For this review, take the finished solid that the model builds, in its own axes (mm). A direction names the side the tool comes from. Give positions to 0.01 mm unless a question says otherwise; leave off trailing zeros. Loops run counter-clockwise (first coordinate to the right, second up) from the corner with the lowest first, then second, coordinate; pieces in that order, holes last. Notation, with made-up numbers: (-5.5, 87.5) - (49.5, 87.5) arc R6 ccw to (49.5, 92.5) - close; hole circle Ø7 at (51, 0). An arc over 180 degrees is marked (long way). Use CSV: the item, a comma, the result in double quotes. Start each with the question number.
1. For faces 1 (the flat face through (-4, -2.704, -9)), 2 (the flat face through (-1, -26.204, -15)), 3 (the cylindrical face through (-25.64, -28.65, -14.79)), list the 3-axis set-ups (+Z, -Z, +X, -X, +Y, -Y) from which the entire face can be reached by the end or side of a thin tool; tool diameter is ignored.
2. Mouldability with a two-part tool opening along Y and no side actions: class faces 4 (the flat face through (-1.8, 3.5, 25)), 5 (the flat face through (-14, 37.796, -2)), 6 (the flat face through (-9, 8.296, 1)) as pulls with the +Y half, pulls with the -Y half, needs draft (parallel to the pull), parting line crosses it, or undercut.
3. Take a section at A-A on z = -5.5. Give the boundary of the cut face in (x, y), plus the area to 3 significant figures.
4. Take a section at D-D on x = -6.5. Give the boundary of the cut face in (y, z), plus the area to 3 significant figures.
5. Wall thickness on line 1 (Y direction, x = -15.5, z = 14.5); line 2 (Y direction, x = -5.5, z = -20.5); line 3 (Z direction, x = -25, y = -14): over which ranges is each line inside the solid? List them lowest first.
6. Take a section at C-C on z = -21.5. Give the boundary of the cut face in (x, y).
7. For pin 1 (3 mm diameter, centred on y = 7.5, z = -11.5, fed in from -X); pin 2 (18.5 mm diameter, centred on y = -7.5, z = 17, fed in from -X); pin 3 (4 mm diameter, centred on x = -23, y = 1, fed in from -Z), all flat-tipped, find the tip position at first contact; note any pin that passes through.
8. Take a section at B-B on y = 4.5. Give the boundary of the cut face in (x, z), plus the area to 3 significant figures.
```python
from build123d import *

# Parameters (mm, degrees)
F0_W      = 28
F0_H      = 69
F1_DEPTH  = 25
F2_T      = -2
F3_R      = 5
F4_R      = 10
F5_W      = 6.9
F5_H      = 11
F6_DEPTH  = 25
F7_W      = 2
F7_H      = 45
F8_DEPTH  = 25
F10_W     = 2
F10_H     = 11
F11_DEPTH = 18
F12_DEPTH = 30


with BuildPart() as f1:
    # F0 (on Top) → F1 (new body)
    with BuildSketch(Plane.XY):
        with Locations((-14.1341709197, 3.2960948795)):
            Rectangle(F0_W, F0_H)
    extrude(amount=F1_DEPTH)

    # F2
    f2_openings = [f1.faces().sort_by_distance(p)[0] for p in [
        (-14.134171, 3.296095, 25),
    ]]
    offset(amount=F2_T, openings=f2_openings)

    # F3
    f3_edges = [f1.edges().sort_by_distance(p)[0] for p in [
        (-0.134171, -31.203905, 12.5),
        (-28.134171, -31.203905, 12.5),
        (-0.134171, 37.796095, 12.5),
        (-28.134171, 37.796095, 12.5),
    ]]
    fillet(f3_edges, radius=F3_R)

    # F4
    f4_edges = [f1.edges().sort_by_distance(p)[0] for p in [
        (-26.134171, 35.796095, 13.5),
        (-26.134171, -29.203905, 13.5),
        (-2.134171, -29.203905, 13.5),
        (-2.134171, 35.796095, 13.5),
    ]]
    fillet(f4_edges, radius=F4_R)

    # F5 (on face) → F6 (cut)
    with BuildSketch(Plane.XY.offset(2)):
        with Locations((-8.5841709197, 2.7960948795)):
            Rectangle(F5_W, F5_H)
    extrude(amount=-F6_DEPTH, mode=Mode.SUBTRACT)

    # F7 (on face) → F8 (cut)
    with BuildSketch(Plane.XY.offset(25)):
        with Locations((-27.1341709197, 3.2960948795)):
            Rectangle(F7_W, F7_H)
    extrude(amount=-F8_DEPTH, mode=Mode.SUBTRACT)

    # F10 (on face) → F11 (join)
    with BuildSketch(Plane(origin=(0, 0, 0), x_dir=(1, 0, 0), z_dir=(0, 0, -1))):
        with Locations((-4.1341709197, -2.7960948795)):
            Rectangle(F10_W, F10_H)
    extrude(amount=F11_DEPTH)

    # F10 (on face) → F12 (join)
    with BuildSketch(Plane(origin=(0, 0, 0), x_dir=(1, 0, 0), z_dir=(0, 0, -1))):
        with BuildLine():
            ThreePointArc((-1.6341702342, -32.7960948795), (-2.6592967008, -35.2709690983), (-5.1341709197, -36.296095565))
            Line((-5.1341709197, -36.296095565), (-23.1341709197, -36.296095565))
            ThreePointArc((-23.1341709197, -36.296095565), (-25.6090451385, -35.2709690983), (-26.6341716051, -32.7960948795))
            Line((-26.6341716051, -32.7960948795), (-26.6341716051, -25.7960948795))
            Line((-26.6341716051, -25.7960948795), (-28.1341709197, -25.7960948795))
            Line((-28.1341709197, -25.7960948795), (-28.1341709197, -32.7960948795))
            ThreePointArc((-28.1341709197, -32.7960948795), (-26.6697048256, -36.3316287854), (-23.1341709197, -37.7960948795))
            Line((-23.1341709197, -37.7960948795), (-5.1341709197, -37.7960948795))
            ThreePointArc((-5.1341709197, -37.7960948795), (-1.5986370137, -36.3316287854), (-0.1341709197, -32.7960948795))
            Line((-0.1341709197, -32.7960948795), (-1.6341702342, -32.7960948795))
        make_face()
        with BuildLine():
            Line((-1.6341709197, 26.2039051205), (-0.1341709197, 26.2039051205))
            ThreePointArc((-0.1341709197, 26.2039051205), (-1.5986370137, 29.7394390264), (-5.1341709197, 31.2039051205))
            Line((-5.1341709197, 31.2039051205), (-23.1341709197, 31.2039051205))
            ThreePointArc((-23.1341709197, 31.2039051205), (-26.6697048256, 29.7394390264), (-28.1341709197, 26.2039051205))
            Line((-28.1341709197, 26.2039051205), (-28.1341709197, 19.2039051205))
            Line((-28.1341709197, 19.2039051205), (-26.6341709197, 19.2039051205))
            Line((-26.6341709197, 19.2039051205), (-26.6341709197, 26.2039051205))
            ThreePointArc((-26.6341709197, 26.2039051205), (-25.6090446538, 28.6787788546), (-23.1341709197, 29.7039051205))
            Line((-23.1341709197, 29.7039051205), (-5.1341709197, 29.7039051205))
            ThreePointArc((-5.1341709197, 29.7039051205), (-2.6592971855, 28.6787788546), (-1.6341709197, 26.2039051205))
        make_face()
    extrude(amount=F12_DEPTH)


solid = f1.part
```
Check result:
1,face 1,"-Z, +X, -X"
1,face 2,"-Z, +X"
1,face 3,"-Z"
2,face 4,"needs draft"
2,face 5,"pulls with the +Y half"
2,face 6,"undercut"
3,outline,"(-28.13, -26.2) arc R5 ccw to (-23.13, -31.2) - (-5.13, -31.2) arc R5 ccw to (-0.13, -26.2) - (-1.63, -26.2) arc R3.5 cw to (-5.13, -29.7) - (-23.13, -29.7) arc R3.5 cw to (-26.63, -26.2) - (-26.63, -19.2) - (-28.13, -19.2) - close; (-28.13, 25.8) - (-26.63, 25.8) - (-26.63, 32.8) arc R3.5 cw to (-23.13, 36.3) - (-5.13, 36.3) arc R3.5 cw to (-1.63, 32.8) - (-0.13, 32.8) arc R5 ccw to (-5.13, 37.8) - (-23.13, 37.8) arc R5 ccw to (-28.13, 32.8) - close; (-5.13, -2.7) - (-3.13, -2.7) - (-3.13, 8.3) - (-5.13, 8.3) - close"
3,area,"137 mm²"
4,outline,"(-31.2, -30) - (-29.7, -30) - (-29.7, 0) - (-2.7, 0) - (-2.7, 2) - (-27.47, 2) - (-27.47, 25) - (-31.2, 25) - close; (8.3, 0) - (36.3, 0) - (36.3, -30) - (37.8, -30) - (37.8, 25) - (34.06, 25) - (34.06, 2) - (8.3, 2) - close"
4,area,"378 mm²"
5,line 1,"y = -31.2 to -29.2, 35.8 to 37.8"
5,line 2,"y = -31.2 to -29.7, 36.3 to 37.8"
5,line 3,"z = 0 to 2"
6,outline,"(-28.13, -26.2) arc R5 ccw to (-23.13, -31.2) - (-5.13, -31.2) arc R5 ccw to (-0.13, -26.2) - (-1.63, -26.2) arc R3.5 cw to (-5.13, -29.7) - (-23.13, -29.7) arc R3.5 cw to (-26.63, -26.2) - (-26.63, -19.2) - (-28.13, -19.2) - close; (-28.13, 25.8) - (-26.63, 25.8) - (-26.63, 32.8) arc R3.5 cw to (-23.13, 36.3) - (-5.13, 36.3) arc R3.5 cw to (-1.63, 32.8) - (-0.13, 32.8) arc R5 ccw to (-5.13, 37.8) - (-23.13, 37.8) arc R5 ccw to (-28.13, 32.8) - close"
7,pin 1,"stops at x = -5.13"
7,pin 2,"stops at x = -2.13"
7,pin 3,"stops at z = 0"
8,outline,"(-26.13, 0) - (-12.03, 0) - (-12.03, 2) - (-26.13, 2) - close; (-5.13, -18) - (-3.13, -18) - (-3.13, 0) - (-0.13, 0) - (-0.13, 25) - (-2.13, 25) - (-2.13, 2) - (-5.13, 2) - close"
8,area,"120 mm²"
